Model file for the job. Use its own axes, mm. Face numbers are marked on the shaded views. A direction names the side the tool comes from. Give positions to 0.01 mm unless a question says otherwise; leave off trailing zeros. Loops run counter-clockwise (first coordinate to the right, second up) from the corner with the lowest first, then second, coordinate; pieces in that order, holes last. Notation, with made-up numbers: (38, 52.5) -> (73, 52.5) arc R16 ccw to (73, 61.5) -> close; hole circle Ø11 at (-3.75, 6). An arc over 180 degrees is marked (long way). Use CSV: the item, a comma, the result in double quotes. Start each with the question number.
(1) 3-axis set-ups, long thin cutter, end or side, ignore diameter. For the marked faces 4, 5 and 6: which of +Z, -Z, +X, -X, +Y, -Y reach the whole face in a straight line?
(2) Cut at D-D on z = -15.5. State how many separate pieces and enclosed holes the cut face has, then the cut area to 3 significant figures.
(3) Cut at B-B on y = 4.75. Write the cut outline in (x, z).
(4) Drill centre lines: probe 1 along Y at (x, z) = (-21, 10.5); probe 2 along Y at (x, z) = (-9.5, -6.5) (3 decimals); probe 3 along X at (y, z) = (4.5, -4.5) (3 decimals). Where is each one in solid material? Low to high.
(5) Flat gauge pins, fed straight in: pin 1 (4 mm diameter, centred on x = 19.5, y = 8.5, fed in from -Z); pin 2 (8 mm diameter, centred on y = 24.5, z = 4, fed in from +X); pin 3 (6.5 mm diameter, centred on x = 0, y = 14.73, fed in from -Z). Where does each tip first touch, or does it go through?
(6) Pull direction Z, two halves, no side cores. Call the marked faces 1, 2 and 3: pulls with the +Z half, pulls with the -Z half, needs draft (parallel to the pull), parting line crosses it, or undercut.
from build123d import *

# Parameters (mm, degrees)
SKETCH1_R               = 22.4
SKETCH1_R_2             = 19
BOSS_EXTRUDE1_DEPTH     = 28
BOSS_EXTRUDE2_DEPTH     = 8.6
SKETCH3_R               = 4
CUT_EXTRUDE1_DEPTH      = 9
SKETCH4_R               = 24.9
SKETCH4_R_2             = 22.3905802
BOSS_EXTRUDE3_DEPTH     = 2
BOSS_EXTRUDE4_START     = -2
SKETCH5_R               = 24.964272213
SKETCH5_R_2             = 22.4
BOSS_EXTRUDE4_DEPTH     = 2
FILLET1_R               = 1
SKETCH7_R               = 1.585
CUT_EXTRUDE2_DEPTH      = 32
SKETCH8_R               = 2.5
CUT_EXTRUDE3_DEPTH      = 3
SKETCH9_R               = 2.5
CUT_EXTRUDE4_DEPTH      = 3
SKETCH10_R              = 2.5
CUT_EXTRUDE5_DEPTH      = 3
MIRROR6_COPY_1_SKETCH_R = 2.5
MIRROR6_COPY_1_DEPTH    = 3
MIRROR6_COPY_2_SKETCH_R = 2.5
MIRROR6_COPY_2_DEPTH    = 3


with BuildPart() as part:
    # Sketch1 → Boss-Extrude1 (new body)
    with BuildSketch(Plane(origin=(0, 0, 0), x_dir=(1, 0, 0), z_dir=(0, 1, 0))):
        with Locations(Location((0, 0, 0), (0, 0, 270))):
            Circle(SKETCH1_R)
        with Locations(Location((0, 0, 0), (0, 0, 270))):
            Circle(SKETCH1_R_2, mode=Mode.SUBTRACT)
    extrude(amount=BOSS_EXTRUDE1_DEPTH)

    # Sketch2 → Boss-Extrude2 (add)
    with BuildSketch(Plane.XZ):
        with BuildLine():
            Line((-22.4, 0), (0, 0))
            Line((0, 0), (22.4, 0))
            ThreePointArc((22.4, 0), (0, -22.4), (-22.4, 0))
        make_face()
    extrude(amount=-BOSS_EXTRUDE2_DEPTH)

    # Sketch3 → Cut-Extrude1 (cut)
    with BuildSketch(Plane(origin=(0, 0, 0), x_dir=(-1, 0, 0), z_dir=(0, -1, 0))):
        Circle(SKETCH3_R)
    extrude(amount=-CUT_EXTRUDE1_DEPTH, mode=Mode.SUBTRACT)

    # Sketch4 → Boss-Extrude3 (add)
    with BuildSketch(Plane(origin=(0, 0, 0), x_dir=(-1, 0, 0), z_dir=(0, -1, 0))):
        with Locations(Location((0, 0, 0), (0, 0, 90))):
            Circle(SKETCH4_R)
        Circle(SKETCH4_R_2, mode=Mode.SUBTRACT)
    extrude(amount=-BOSS_EXTRUDE3_DEPTH)

    # Sketch5 → Boss-Extrude4 (add)
    with BuildSketch(Plane(origin=(0, 28, 0), x_dir=(1, 0, 0), z_dir=(0, 1, 0)).offset(BOSS_EXTRUDE4_START)):
        with Locations(Location((0, 0, 0), (0, 0, 270))):
            Circle(SKETCH5_R)
        with Locations(Location((0, 0, 0), (0, 0, 90))):
            Circle(SKETCH5_R_2, mode=Mode.SUBTRACT)
    extrude(amount=BOSS_EXTRUDE4_DEPTH)

    # Fillet1
    fillet1_edges = [part.edges().sort_by_distance(p)[0] for p in [
        (0, 2, -22.4),
        (0, 26, -22.4),
    ]]
    fillet(fillet1_edges, radius=FILLET1_R)

    # Sketch7 → Cut-Extrude2 (cut)
    with BuildSketch(Plane.XY.offset(-25)):
        with Locations(Location((-9.5, 4.5, 0), (0, 0, 251.150810429))):
            Circle(SKETCH7_R)
    cut_extrude2 = extrude(amount=CUT_EXTRUDE2_DEPTH, mode=Mode.SUBTRACT)

    # Mirror1: Cut-Extrude2 across plane
    add(cut_extrude2.mirror(Plane(origin=(0, 0, 0), x_dir=(0, 0, 1), z_dir=(1, 0, 0))), mode=Mode.SUBTRACT)

    # Sketch8 → Cut-Extrude3 (cut)
    with BuildSketch(Plane.XY.offset(-25)):
        with Locations(Location((0, 14.732501926, 0), (0, 0, 90))):
            Circle(SKETCH8_R)
    cut_extrude3 = extrude(amount=CUT_EXTRUDE3_DEPTH, mode=Mode.SUBTRACT)

    # Mirror2: Cut-Extrude3 across plane
    add(cut_extrude3.mirror(Plane.XY), mode=Mode.SUBTRACT)

    # Sketch9 → Cut-Extrude4 (cut)
    with BuildSketch(Plane(origin=(25, 0, 0), x_dir=(0, 0, -1), z_dir=(1, 0, 0))):
        with Locations((0, 14.732501926)):
            Circle(SKETCH9_R)
    cut_extrude4 = extrude(amount=-CUT_EXTRUDE4_DEPTH, mode=Mode.SUBTRACT)

    # Mirror3: Cut-Extrude4 across plane
    add(cut_extrude4.mirror(Plane(origin=(0, 0, 0), x_dir=(0, 0, 1), z_dir=(1, 0, 0))), mode=Mode.SUBTRACT)

    # Sketch10 → Cut-Extrude5 (cut)
    with BuildSketch(Plane(origin=(17.67766953, 0, -17.67766953), x_dir=(-0.7071067811865477, 0, -0.7071067811865475), z_dir=(0.7071067811865475, 0, -0.7071067811865477))):
        with Locations((-0.521742336, 14.830490085)):
            Circle(SKETCH10_R)
    cut_extrude5 = extrude(amount=-CUT_EXTRUDE5_DEPTH, mode=Mode.SUBTRACT)

    # Mirror4: Cut-Extrude5 across plane
    add(cut_extrude5.mirror(Plane(origin=(0, 0, 0), x_dir=(0.7071067811865478, 0, 0.7071067811865472), z_dir=(0.7071067811865475, 0, -0.7071067811865477))), mode=Mode.SUBTRACT)

    # Mirror5: Cut-Extrude5 across plane
    add(cut_extrude5.mirror(Plane(origin=(0, 0, 0), x_dir=(0, 0, 1), z_dir=(1, 0, 0))), mode=Mode.SUBTRACT)

    # Mirror6 copy 1 sketch → Mirror6 copy 1 (cut)
    with BuildSketch(Plane(origin=(17.67766953, 0, 17.67766953), x_dir=(0.7071067811865477, 0, -0.7071067811865475), z_dir=(0.7071067811865477, 0, 0.7071067811865479))):
        with Locations((-0.521742336, 14.830490085)):
            Circle(MIRROR6_COPY_1_SKETCH_R)
    extrude(amount=-MIRROR6_COPY_1_DEPTH, mode=Mode.SUBTRACT)

    # Mirror6 copy 2 sketch → Mirror6 copy 2 (cut)
    with BuildSketch(Plane(origin=(-17.67766953, 0, -17.67766953), x_dir=(0.7071067811865477, 0, -0.7071067811865475), z_dir=(-0.7071067811865475, 0, -0.7071067811865477))):
        with Locations((-0.521742336, -14.830490085)):
            Circle(MIRROR6_COPY_2_SKETCH_R)
    extrude(amount=-MIRROR6_COPY_2_DEPTH, mode=Mode.SUBTRACT)


solid = part.part
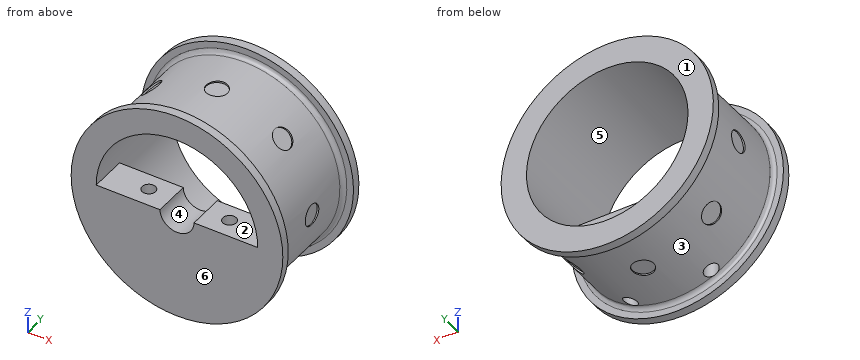
Check result:
1,face 4,"+Y, -Y"
1,face 5,"+Y"
1,face 6,"+Z, -Z, +X, -X, -Y"
2,separate pieces,"1"
2,enclosed holes,"2"
2,area,"486 mm²"
3,outline,"(-19, 0) arc R19 cw to (19, 0) -> (11.07, 0) -> (11.07, -19.48) arc R22.4 ccw (long way) to (-11.07, -19.48) -> (-11.07, 0) -> close; (-7.93, -20.95) arc R22.4 ccw to (7.93, -20.95) -> (7.93, 0) -> (4, 0) arc R4 cw to (-4, 0) -> (-7.93, 0) -> close"
4,probe 1,"0 to 2, 26 to 28"
4,probe 2,"0 to 2.915, 6.085 to 8.6"
4,probe 3,"-21.943 to -11.085, -7.915 to 7.915, 11.085 to 21.943"
5,pin 1,"z = -13.98"
5,pin 2,"x = 24.96"
5,pin 3,"z = -22.4"
6,face 1,"needs draft"
6,face 2,"undercut"
6,face 3,"parting line crosses it"
